from build123d import *

# Parameters (mm, degrees)
F1_DEPTH       = 1200
F2_R           = 8
F4_D           = 3
F4_CSINK_D     = 10
F4_CSINK_ANGLE = 90


with BuildPart() as f1:
    # F0 (on Front) → F1 (new body)
    with BuildSketch(Plane.XZ):
        with BuildLine():
            Line((7, 80), (0, 80))
            Line((0, 80), (0, 3.428398))
            ThreePointArc((0, 3.428398), (-0.876289, 0.600854), (-3.198004, -1.235592))
            Line((-3.198004, -1.235592), (-220, -85))
            Line((-220, -85), (-217.477205, -91.529587))
            Line((-217.477205, -91.529587), (-0.675209, -7.765179))
            ThreePointArc((-0.675209, -7.765179), (4.896906, -3.357709), (7, 3.428398))
            Line((7, 3.428398), (7, 80))
        make_face()
    extrude(amount=F1_DEPTH)

    # F2
    f2_edges = [f1.edges().sort_by_distance(p)[0] for p in [
        (3.5, -1200, 80),
        (3.5, 0, 80),
        (-218.738603, 0, -88.264793),
        (-218.738603, -1200, -88.264793),
    ]]
    fillet(f2_edges, radius=F2_R)

    # F4 (through all)
    with Locations(Plane.YZ.offset(7)):
        with Locations((-900, 41.714199), (-1050, 41.714199), (-750, 41.714199), (-600, 41.714199), (-450, 41.714199), (-300, 41.714199), (-150, 41.714199)):
            CounterSinkHole(F4_D / 2, F4_CSINK_D / 2, counter_sink_angle=F4_CSINK_ANGLE)


solid = f1.part
Input: part model. Units: mm. Frame: model coordinates. A direction names the side the tool comes from. Round coordinates to 2 decimals unless told otherwise and drop trailing zeros. Write each loop counter-clockwise with the first axis right and the second up, starting at its lowest first coordinate (ties: lowest second). Pieces come first, ordered by that corner, then holes.
1) Cut plane A-A (y = -184.5). Return the cut outline in (x, z).
2) Cut plane C-C (x = -169.5). Return the cut outline in (y, z).
3) Contact query for flat-ended pins moving along their axis: P1, Ø6, axis at x = -86, y = -685, coming from the +Z side; P2, Ø2.5, axis at y = -600, z = 41.71, coming from the -X side; P3, Ø5, axis at y = -900, z = 41.71, coming from the -X side; P4, Ø3.5, axis at y = -300, z = 41.71, coming from the +X side. Output: stop coordinate, or through.
4) Reachability of faces 1 (the flat face through (0, -592, 42)), 2 (the flat face through (-110.594, -591.6, -50.234)) from +Z, -Z, +X, -X, +Y, -Y: full face, straight path, thin tool, end or side. Return the list, or none.
5) Cut plane B-B (z = 61). Return the cut outline in (x, y), then the cut area to 3 significant figures.
6) Ray query, L1, parallel to X at y = -993, z = 24.5; L2, parallel to Z at x = 2, y = -900; L3, parallel to Z at x = 1.65, y = -450. Return the intervals inside material, ascending.
Geometry says:
1. outline: (-220, -85) - (-217.48, -91.53) - (-0.68, -7.77) arc R12 ccw to (7, 3.43) - (7, 80) - (0, 80) - (0, 3.43) arc R5 cw to (-3.2, -1.24) - close
2. outline: (-1200, -72.99) - (0, -72.99) - (0, -65.49) - (-1200, -65.49) - close
3. P1: stops at z = -32.07
3. P2: passes through
3. P3: stops at x = 0
3. P4: stops at x = 3.75
4. face 1: +Z, -X, +Y, -Y
4. face 2: -Z, +X, +Y, -Y
5. outline: (0, -1200) - (7, -1200) - (7, 0) - (0, 0) - close
5. area: 8,400 mm2
6. L1: x = 0 to 7
6. L2: z = -6.32 to 40.21, 43.21 to 80
6. L3: z = -6.56 to 40.21, 43.21 to 80
